Model file for the job. Use its own axes, mm. Face numbers are marked on the shaded views. A direction names the side the tool comes from. Coordinates: 2 decimals unless noted, no trailing zeros. Write each loop counter-clockwise with the first axis right and the second up, starting at its lowest first coordinate (ties: lowest second). Pieces come first, ordered by that corner, then holes. Notation, with made-up numbers: M 27.5,-4.75 L 53.5,-4.75 A16 ccw 53.5,26.25 Z; hole C -32,64 d8. An arc over 180 degrees is marked long. Answer in a Markdown table with one row per item. Add a question column.
```python
from build123d import *

# Parameters (mm, degrees)
SKETCH1_R                = 29
BOSS_EXTRUDE1_DEPTH      = 2.5
SKETCH3_W                = 8
SKETCH3_H                = 5
BOSS_EXTRUDE2_DEPTH      = 31.5
SKETCH5_R                = 1.4
CUT_EXTRUDE1_DEPTH       = 44.107423955
FILLET2_R                = 1.5
CIRPATTERN1_COUNT        = 4
FILLET2_OF_CIRPATTERN1_R = 1.5
SKETCH6_R                = 3.9
CUT_EXTRUDE2_DEPTH       = 45.827446949
SKETCH7_W                = 5.5
SKETCH7_H                = 10.6
CUT_EXTRUDE3_DEPTH       = 45.827446949
SKETCH8_R                = 2.05
CUT_EXTRUDE4_DEPTH       = 45.827446949
SKETCH9_R                = 3.75
CUT_EXTRUDE5_DEPTH       = 3


with BuildPart() as part:
    # Sketch1 → Boss-Extrude1 (new, symmetric)
    with BuildSketch(Plane(origin=(0, 0, 0), x_dir=(1, 0, 0), z_dir=(0, 1, 0))):
        with Locations(Location((0, 0, 0), (0, 0, 270))):
            Circle(SKETCH1_R)
    extrude(amount=BOSS_EXTRUDE1_DEPTH, both=True)

    # Sketch3 → Boss-Extrude2 (add)
    with BuildSketch(Plane.XY):
        Rectangle(SKETCH3_W, SKETCH3_H)
    boss_extrude2 = extrude(amount=BOSS_EXTRUDE2_DEPTH)

    # Sketch5 → Cut-Extrude1 (cut, through all)
    with BuildSketch(Plane(origin=(0, 2.5, 0), x_dir=(1, 0, 0), z_dir=(0, 1, 0))):
        with Locations(Location((0, -28.3, 0), (0, 0, 270))):
            Circle(SKETCH5_R)
    cut_extrude1 = extrude(amount=-CUT_EXTRUDE1_DEPTH, mode=Mode.SUBTRACT)

    # Fillet2
    fillet2_edges = [part.edges().sort_by_distance(p)[0] for p in [
        (4, 0, 28.722813233),
        (-4, 0, 28.722813233),
        (-4, 0, 31.5),
        (4, 0, 31.5),
    ]]
    fillet(fillet2_edges, radius=FILLET2_R - 0.0001)  # a hair under: the kernel refuses the full size

    # CirPattern1: Boss-Extrude2, Cut-Extrude1 ×4 about axis
    cirpattern1_axis = Axis((0, 0, 0), (0, 1, 0))
    add([boss_extrude2.rotate(cirpattern1_axis, i * 360 / CIRPATTERN1_COUNT) for i in range(1, CIRPATTERN1_COUNT)])
    add([cut_extrude1.rotate(cirpattern1_axis, i * 360 / CIRPATTERN1_COUNT) for i in range(1, CIRPATTERN1_COUNT)], mode=Mode.SUBTRACT)

    # Fillet2 of CirPattern1
    fillet2_of_cirpattern1_edges = [part.edges().sort_by_distance(p)[0] for p in [
        (28.722813233, 0, -4),
        (28.722813233, 0, 4),
        (31.5, 0, 4),
        (31.5, 0, -4),
        (-4, 0, -28.722813233),
        (4, 0, -28.722813233),
        (4, 0, -31.5),
        (-4, 0, -31.5),
        (-28.722813233, 0, 4),
        (-28.722813233, 0, -4),
        (-31.5, 0, -4),
        (-31.5, 0, 4),
    ]]
    fillet(fillet2_of_cirpattern1_edges, radius=FILLET2_OF_CIRPATTERN1_R - 0.0001)  # a hair under: the kernel refuses the full size

    # Sketch6 → Cut-Extrude2 (cut, through all)
    with BuildSketch(Plane(origin=(0, 2.5, 0), x_dir=(1, 0, 0), z_dir=(0, 1, 0))):
        with Locations(Location((-19, 0, 0), (0, 0, 270))):
            Circle(SKETCH6_R)
    extrude(amount=-CUT_EXTRUDE2_DEPTH, mode=Mode.SUBTRACT)

    # Sketch7 → Cut-Extrude3 (cut, through all)
    with BuildSketch(Plane(origin=(0, 2.5, 0), x_dir=(1, 0, 0), z_dir=(0, 1, 0))):
        with Locations((-16.15, 11.6)):
            Rectangle(SKETCH7_W, SKETCH7_H)
    extrude(amount=-CUT_EXTRUDE3_DEPTH, mode=Mode.SUBTRACT)

    # Sketch8 → Cut-Extrude4 (cut, through all)
    with BuildSketch(Plane.XZ.offset(2.5)):
        with Locations(Location((0.80857407, -17.981829939, 0), (0, 0, 270))):
            Circle(SKETCH8_R)
        with Locations(Location((16.569087362, 7.033160313, 0), (0, 0, 270))):
            Circle(SKETCH8_R)
        with Locations(Location((-12.373363213, 13.072868194, 0), (0, 0, 270))):
            Circle(SKETCH8_R)
    extrude(amount=-CUT_EXTRUDE4_DEPTH, mode=Mode.SUBTRACT)

    # Sketch9 → Cut-Extrude5 (cut)
    with BuildSketch(Plane(origin=(0, -2.5, 0), x_dir=(-1, 0, 0), z_dir=(0, -1, 0))):
        with Locations(Location((-0.80857407, 17.981829939, 0), (0, 0, 90))):
            Circle(SKETCH9_R)
        with Locations(Location((12.373363213, -13.072868194, 0), (0, 0, 90))):
            Circle(SKETCH9_R)
        with Locations(Location((-16.569087362, -7.033160313, 0), (0, 0, 90))):
            Circle(SKETCH9_R)
    extrude(amount=-CUT_EXTRUDE5_DEPTH, mode=Mode.SUBTRACT)


solid = part.part
```
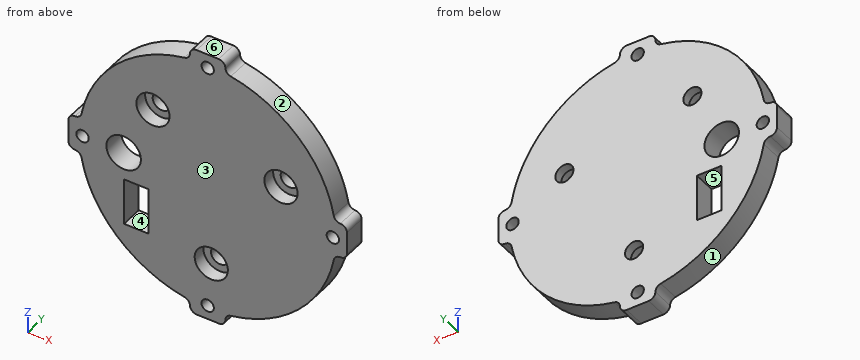
1) Flat gauge pins, fed straight in: pin 1 Ø2 at (x, z) = (18.5, 5.5) entering from -Y; pin 2 Ø1 at (x, y) = (19.5, -0.5) entering from +Z; pin 3 Ø1 at (x, y) = (15.5, 1.5) entering from -Z; pin 4 Ø6 at (x, z) = (-19, 0) entering from +Y. Where does each tip first touch, or does it go through?
2) Two-plate mould, pull along X, no slides. Class the marked faces 1, 2, 3 and 4: released by +X, released by -X, zero draft, split by the parting line, or undercut.
3) Slice it at C-C (z = -18.5). Give the cut face in (x, y), then the cut area to 3 significant figures.
4) Slice it at A-A (z = 0). Give the cut face in (x, y).
5) Drill centre lines: probe 1 along Z at (x, y) = (-18.5, -1.5); probe 2 along X at (y, z) = (-1.1, -20); probe 3 along X at (y, z) = (-1.5, 7). Where is each one in solid material? Low to high.
6) Slice it at D-D (z = 13.5). Give the cut face in (x, y).
7) Which spindle directions (+Z, -Z, +X, -X, +Y, -Y) get a long thin tool onto all of the face, cutting with end or side? Do the marked faces 5 and 6. Say none if no direction does.
8) Slice it at B-B (x = -17). Give the cut face in (y, z).
Ans:
| question | item | result |
|---|---|---|
| 1 | pin 1 | stops at y = 0.5 |
| 1 | pin 2 | stops at z = 21.91 |
| 1 | pin 3 | stops at z = -24.82 |
| 1 | pin 4 | passes through |
| 2 | face 1 | released by -X |
| 2 | face 2 | released by +X |
| 2 | face 3 | zero draft |
| 2 | face 4 | undercut |
| 3 | outline | M -22.33,-2.5 L -2.91,-2.5 L -2.91,0.5 L -1.17,0.5 L -1.17,2.5 L -22.33,2.5 Z; M 2.79,0.5 L 4.52,0.5 L 4.52,-2.5 L 22.33,-2.5 L 22.33,2.5 L 2.79,2.5 Z |
| 3 | area | 193 mm2 |
| 4 | outline | M -31.5,-2.5 L -29.7,-2.5 L -29.7,2.5 L -31.5,2.5 Z; M -26.9,-2.5 L -22.9,-2.5 L -22.9,2.5 L -26.9,2.5 Z; M -15.1,-2.5 L 26.9,-2.5 L 26.9,2.5 L -15.1,2.5 Z; M 29.7,-2.5 L 31.5,-2.5 L 31.5,2.5 L 29.7,2.5 Z |
| 5 | probe 1 | z = -22.33 to -16.9, -6.3 to -3.87, 3.87 to 22.33 |
| 5 | probe 2 | x = -21 to -2.35, 3.97 to 21 |
| 5 | probe 3 | x = -28.14 to 12.82, 20.32 to 28.14 |
| 6 | outline | M -25.67,-2.5 L -16.1,-2.5 L -16.1,0.5 L -14.38,0.5 L -14.38,2.5 L -25.67,2.5 Z; M -10.37,0.5 L -8.65,0.5 L -8.65,-2.5 L 25.67,-2.5 L 25.67,2.5 L -10.37,2.5 Z |
| 7 | face 5 | +Y, -Y |
| 7 | face 6 | +Z, +X, -X, +Y, -Y |
| 8 | outline | M -2.5,-23.49 L 2.5,-23.49 L 2.5,-16.9 L -2.5,-16.9 Z; M -2.5,-6.3 L 2.5,-6.3 L 2.5,-3.35 L -2.5,-3.35 Z; M -2.5,3.35 L 2.5,3.35 L 2.5,23.49 L -2.5,23.49 Z |
